Verification items for the finished model (mm, model axes). A direction names the side the tool comes from. Round coordinates to 2 decimals unless told otherwise and drop trailing zeros. Write each loop counter-clockwise with the first axis right and the second up, starting at its lowest first coordinate (ties: lowest second). Pieces come first, ordered by that corner, then holes. Notation, with made-up numbers: (32, 74) - (81, 74) arc R33 cw to (81, 110) - close; hole circle Ø4 at (-39, 89). An arc over 180 degrees is marked (long way). Answer as a JSON object with one key per item and string values.
Autodesk Inventor part; units mm, degrees
ref_plane "YZ Plane" through (0, 0, 0) normal (1, 0, 0) x (0, 1, 0)
ref_plane "XZ Plane" through (0, 0, 0) normal (0, 1, 0) x (-1, 0, 0)
ref_plane "XY Plane" through (0, 0, 0) normal (0, 0, 1) x (1, 0, 0)
sketch "Sketch1" plane through (0, 0, 0) normal (0, 1, 0) x (-1, 0, 0)
  line L0 (0, 0) -> (22.3, 0)
  line L1 (22.3, 0) -> (22.3, -22.3)
  line L2 (22.3, -22.3) -> (0, -22.3)
  line L3 (0, -22.3) -> (0, 0)
  dimension "d0" = 22.3
  dimension "d1" = 22.3
extrude "Extrusion1" add sketch "Sketch1" along normal blind 3
ref_plane "Work Plane1" through (-11.15, 0, 0) normal (1, 0, 0) x (0, 0, -1)
sketch "Sketch3" plane through (-11.15, 0, 0) normal (1, 0, 0) x (0, 0, -1)
  line L0 (0, 3) -> (22.3, 3)
  circle A0 centre (11.15, 8) radius 2.5
  arc A1 (13.8913, 10.913) -> (8.4087, 10.913) centre (11.15, 8) ccw
  line L1 (0, 0) -> (0, 3)
  line L2 (0, 3) -> (8.4087, 10.913)
  line L3 (13.8913, 10.913) -> (22.3, 3)
  dimension "d5" = 5
  dimension "d6" = 8
  dimension "d7" = 11.15
  dimension "d8" = 5
extrude "Extrusion2" add sketch "Sketch3" along normal mid plane 5
chamfer "Chamfer1" distance 1 angle 45 1 edges at (-8.65, 3, -11.15)
chamfer "Chamfer2" distance 1 angle 45 1 edges at (-13.65, 3, -11.15)
chamfer "Chamfer3" distance 1 angle 45 3 edges at (-13.65, 12, -11.15) (-13.65, 7.4565, -17.5643) (-13.65, 7.4565, -4.7357)
chamfer "Chamfer4" distance 1 angle 45 3 edges at (-8.65, 7.4565, -4.7357) (-8.65, 12, -11.15) (-8.65, 7.4565, -17.5643)
chamfer "Chamfer5" distance 1 angle 45 10 edges at (-18.475, 3, 0) (-22.3, 3, -11.15) (-3.825, 3, 0) (0, 3, -11.15) (-3.825, 3, -22.3) (-18.475, 3, -22.3) (0, 1.5, -22.3) (0, 1.5, 0) (-22.3, 1.5, -22.3) (-22.3, 1.5, 0)
chamfer "Chamfer6" distance 1 angle 45 2 edges at (-7.15, 2.5, 0) (-15.15, 2.5, 0)
chamfer "Chamfer7" distance 1 angle 45 2 edges at (-7.15, 2.5, -22.3) (-15.15, 2.5, -22.3)
equation "\"d1\" = d0"
equation "\"d7\" = 0.5 * d0"
equation "\"d4\" = -0.5 * d0"
properties part number "TrackPivotConnector"
Q1. Section check B-B, the plane z = -11.15. Record the cut outline in (x, y), then the cut area to 3 significant figures.
Geometry check:
{"outline": "(-22.3, 0) - (0, 0) - (0, 2) - (-1, 3) - (-7.65, 3) - (-8.65, 4) - (-8.65, 5.5) - (-13.65, 5.5) - (-13.65, 4) - (-14.65, 3) - (-21.3, 3) - (-22.3, 2) - close; (-13.65, 10.5) - (-8.65, 10.5) - (-8.65, 11) - (-9.65, 12) - (-12.65, 12) - (-13.65, 11) - close", "area": "85.9 mm2"}
Q2. Gauge pin test, flat ends, axial feed: P1, Ø2, axis at x = -18.5, z = -12.5, coming from the +Y side; P2, Ø4, axis at y = 4.5, z = -9.5, coming from the -X side. Record the tip position at first contact, or that the pin passes through.
Geometry check:
{"P1": "stops at y = 3", "P2": "stops at x = -21.8"}
Q3. Set-up check for faces 1 (the flat face through (-4.6, 2.5, -0.5)), 2 (the flat face through (-13.65, 5, -11)), 3 (the flat face through (-17.8, 2.5, -21.8)), 4 (the flat face through (-11, 0, -11)): record each of +Z, -Z, +X, -X, +Y, -Y from which the full face is reachable in a straight line by a thin tool's end or side.
Geometry check:
{"face 1": "+Z, +X, +Y", "face 2": "+Z, -Z, -X, +Y", "face 3": "-Z, -X, +Y", "face 4": "+Z, -Z, +X, -X, -Y"}
Q4. Material ranges on line 1 along Y through (x, z) = (-9.7, -11.15); line 2 along X through (y, z) = (6.75, -17.5); line 3 along X through (y, z) = (6.5, -14.75), recorded low to high. Write a range as [from, to].
Geometry check:
{"line 1": "y = [0, 5.5], [10.5, 12]", "line 2": "x = [-13.21, -9.09]", "line 3": "x = [-13.65, -8.65]"}
Q5. Section check D-D, the plane x = -7.25. Record the cut outline in (y, z).
Geometry check:
{"outline": "(0, -22.3) - (2, -22.3) - (3, -21.3) - (3, -1) - (2, 0) - (0, 0) - close"}
Q6. Section check C-C, the plane y = 8. Record the cut outline in (x, z), then the cut area to 3 significant figures.
Geometry check:
{"outline": "(-13.65, -15.53) - (-12.65, -16.99) - (-9.65, -16.99) - (-8.65, -15.53) - (-8.65, -13.65) - (-13.65, -13.65) - close; (-13.65, -8.65) - (-8.65, -8.65) - (-8.65, -6.77) - (-9.65, -5.31) - (-12.65, -5.31) - (-13.65, -6.77) - close", "area": "30.4 mm2"}
Q7. Section check A-A, the plane x = -11. Record the cut outline in (y, z), then the cut area to 3 significant figures.
Geometry check:
{"outline": "(0, -22.3) - (3, -22.3) - (10.91, -13.89) arc R4 ccw to (10.91, -8.41) - (3, 0) - (0, 0) - close; hole circle Ø5 at (8, -11.15)", "area": "161 mm2"}
